```python
from build123d import *

# Parameters (mm, degrees)
SKETCH2_R               = 75
BOSS_EXTRUDE1_DEPTH     = 85
SKETCH4_R               = 65
CUT_EXTRUDE2_DEPTH      = 25
SKETCH5_R               = 55
CUT_EXTRUDE3_DEPTH      = 50
SKETCH7_R               = 2.5
CUT_EXTRUDE4_DEPTH      = 20
CIRPATTERN1_COUNT       = 5
BOSS_EXTRUDE2_DEPTH     = 85
CUT_EXTRUDE9_DEPTH      = 222.85434026
CUT_EXTRUDE9_DEPTH_BACK = 45
SKETCH29_W              = 52.076433836
SKETCH29_H              = 20
SKETCH23_R              = 7.5
CUT_EXTRUDE8_DEPTH      = 176.561799548
BOSS_EXTRUDE4_DEPTH     = 10
BOSS_EXTRUDE5_DEPTH     = 10
SKETCH32_R              = 5
CUT_EXTRUDE10_DEPTH     = 10


with BuildPart() as part:
    # Sketch2 → Boss-Extrude1 (new body)
    with BuildSketch(Plane(origin=(0, 0, 0), x_dir=(0, 1, 0), z_dir=(0, 0, 1))):
        with Locations(Location((0, 0, 0), (0, 0, 270))):
            Circle(SKETCH2_R)
    extrude(amount=BOSS_EXTRUDE1_DEPTH)

    # Sketch4 → Cut-Extrude2 (cut)
    with BuildSketch(Plane.XY.offset(85)):
        Circle(SKETCH4_R)
    extrude(amount=-CUT_EXTRUDE2_DEPTH, mode=Mode.SUBTRACT)

    # Sketch5 → Cut-Extrude3 (cut)
    with BuildSketch(Plane.XY.offset(60)):
        Circle(SKETCH5_R)
    extrude(amount=-CUT_EXTRUDE3_DEPTH, mode=Mode.SUBTRACT)

    # Sketch7 → Cut-Extrude4 (cut)
    with BuildSketch(Plane.XY.offset(85)):
        with Locations((0, 69.72339814)):
            Circle(SKETCH7_R)
    cut_extrude4 = extrude(amount=-CUT_EXTRUDE4_DEPTH, mode=Mode.SUBTRACT)

    # CirPattern1: Cut-Extrude4 ×5 about axis
    cirpattern1_axis = Axis((0, 0, 0), (0, 0, 1))
    for i in range(1, CIRPATTERN1_COUNT):
        add(cut_extrude4.rotate(cirpattern1_axis, i * 360 / CIRPATTERN1_COUNT), mode=Mode.SUBTRACT)

    # Sketch15 → Boss-Extrude2 (add)
    with BuildSketch(Plane(origin=(0, 0, 0), x_dir=(1, 0, 0), z_dir=(0, 0, -1))):
        Polygon((0, 70.334993138), (26.038216918, 70.334993138), (26.038216918, 115.707494064), (-26.038216918, 115.707494064), (-26.038216918, 70.334993138), align=None)
    extrude(amount=-BOSS_EXTRUDE2_DEPTH)

    # Sketch29 → Cut-Extrude9 (cut, two sides: drawn at the far end of the back side and taken through both)
    with BuildSketch(Plane.XZ.offset(115.707494064).offset(-CUT_EXTRUDE9_DEPTH_BACK)):
        with Locations((0, 75)):
            Rectangle(SKETCH29_W, SKETCH29_H)
        with Locations((0, 10)):
            Rectangle(SKETCH29_W, SKETCH29_H)
    extrude(amount=CUT_EXTRUDE9_DEPTH + CUT_EXTRUDE9_DEPTH_BACK, mode=Mode.SUBTRACT)

    # Sketch23 → Cut-Extrude8 (cut, through all)
    with BuildSketch(Plane(origin=(-26.038216918, 0, 0), x_dir=(0, -1, 0), z_dir=(-1, 0, 0))):
        with Locations((90.556929386, 51.29930896)):
            Circle(SKETCH23_R)
        with Locations((90.556929386, 32.361665764)):
            Circle(SKETCH23_R)
    extrude(amount=-CUT_EXTRUDE8_DEPTH, mode=Mode.SUBTRACT)

    # Sketch30 → Boss-Extrude4 (add)
    with BuildSketch(Plane(origin=(0, 0, 0), x_dir=(1, 0, 0), z_dir=(0, 0, -1))):
        with BuildLine():
            Line((-91.060110116, 13.313174206), (91.197550371, 13.313174206))
            ThreePointArc((91.197550371, 13.313174206), (104.510724577, 0), (91.197550371, -13.313174206))
            Line((91.197550371, -13.313174206), (-91.060110116, -13.313174206))
            ThreePointArc((-91.060110116, -13.313174206), (-104.373284322, 0), (-91.060110116, 13.313174206))
        make_face()
    extrude(amount=-BOSS_EXTRUDE4_DEPTH)

    # Sketch31 → Boss-Extrude5 (add)
    with BuildSketch(Plane(origin=(0, 0, 0), x_dir=(1, 0, 0), z_dir=(0, 0, -1))):
        with BuildLine():
            Line((12.768161156, -41.533975832), (12.768161156, -98.589265102))
            ThreePointArc((12.768161156, -98.589265102), (0, -111.357426258), (-12.768161156, -98.589265102))
            Line((-12.768161156, -98.589265102), (-12.768161156, -41.533975832))
            ThreePointArc((-12.768161156, -41.533975832), (0, -28.765814675), (12.768161156, -41.533975832))
        make_face()
    extrude(amount=-BOSS_EXTRUDE5_DEPTH)

    # Sketch32 → Cut-Extrude10 (cut)
    with BuildSketch(Plane.XY.offset(10)):
        with Locations((-89.533828586, 0)):
            Circle(SKETCH32_R)
        with Locations((0, 96.564616818)):
            Circle(SKETCH32_R)
        with Locations((89.966014067, 0)):
            Circle(SKETCH32_R)
    extrude(amount=-CUT_EXTRUDE10_DEPTH, mode=Mode.SUBTRACT)


solid = part.part
```
The listing builds one solid part. Answer for the finished solid, in the listing's coordinates (mm). A direction names the side the tool comes from. Coordinates: 2 decimals unless noted, no trailing zeros. Order: outer loops, then holes, each group sorted by start corner. A loop starts at its lowest first (then second) coordinate and runs counter-clockwise, first axis right, second up. Notation, with made-up numbers: M -22.75,79 L 31.25,79 A15 cw 31.25,106 Z; hole C 89,19.25 d2. An arc over 180 degrees is marked long. Answer as a JSON object with one key per item and string values. Group by question number.
1. Section C-C on x = 46.5 is taken. Write down the section's boundary in (y, z).
2. Determine the mould class of faces 5 (the flat face through (-82, 13.313, 5)), 6 (the cylindrical face through (-68.49, 20.32, 75.14)), 7 (the flat face through (0, 88, 10)) for opening direction Y: released by +Y, released by -Y, zero draft, split by the parting line, or undercut.
3. Straight lines are drawn through the part: line 1 (Y direction, x = 0, z = 32); line 2 (Y direction, x = 0, z = 75); line 3 (X direction, y = 23.5, z = 14.5). For each, find the intervals that lie inside material, in ascending order.
4. A tool of negligible diameter and unlimited length cuts with its end or side. For faces 1 (the flat face through (-1, 1, 10)), 2 (the flat face through (26.038, -93, 42)), 3 (the flat face through (12.768, 86, 5)), 4 (the flat face through (0, -93, 20)), from which of +Z, -Z, +X, -X, +Y, -Y can it reach the whole face along a straight path? Write none if from no direction.
5. Flat-ended cylindrical pins translate along their axes: P1, Ø6, axis at y = -67.5, z = 39.5, coming from the -X side; P2, Ø13.5, axis at y = -87.5, z = 57.5, coming from the -X side; P3, Ø3, axis at y = 47.5, z = 55.5, coming from the -X side. Find the tip coordinate at first contact, or state that the pin passes through.
6. Section A-A on y = 0 is taken. Write down the section's boundary in (x, z), then the cut area to 3 significant figures.
7. Section D-D on z = 69 is taken. State how many separate pieces and enclosed holes the cut face has, then the cut area to 3 significant figures.
8. Section B-B on z = 55 is taken. Write down the section's boundary in (x, y) (1 decimal), then the cut area to 3 significant figures.
Values follow:
{
 "1": {"outline": "M -58.85,0 L 58.85,0 L 58.85,85 L 45.42,85 L 45.42,60 L 29.37,60 L 29.37,10 L -29.37,10 L -29.37,60 L -45.42,60 L -45.42,85 L -58.85,85 Z"},
 "2": {"face 5": "released by +Y", "face 6": "undercut", "face 7": "zero draft"},
 "3": {"line 1": "-115.71 to -98.05, -83.07 to -55, 55 to 75", "line 2": "-70.71 to -65, 65 to 67.22, 72.22 to 75", "line 3": "-71.22 to -49.73, 49.73 to 71.22"},
 "4": {"face 1": "+Z", "face 2": "+Z, -Z, +X, -Y", "face 3": "+Z, -Z, +X, +Y", "face 4": "-Z, +X, -X, -Y"},
 "5": {"P1": "x = -38.27", "P2": "x = -26.04", "P3": "x = -59.24"},
 "6": {"outline": "M -104.37,0 L -94.53,0 L -94.53,10 L -104.37,10 Z; M -84.53,0 L 84.97,0 L 84.97,10 L 75,10 L 75,85 L 65,85 L 65,60 L 55,60 L 55,10 L -55,10 L -55,60 L -65,60 L -65,85 L -75,85 L -75,10 L -84.53,10 Z; M 94.97,0 L 104.51,0 L 104.51,10 L 94.97,10 Z", "area": "4,390 mm2"},
 "7": {"separate pieces": "1", "enclosed holes": "6", "area": "4,160 mm2"},
 "8": {"outline": "M -26,-115.7 L 26,-115.7 L 26,-97.1 L -26,-97.1 Z; M -26,-84 L 26,-84 L 26,-70.3 A75 ccw long -26,-70.3 Z; hole C 0,0 d110", "area": "9,690 mm2"}
}
